Design review of the part shown in the three views and the two pictorial views. Dimensions are in mm from the part's minimum x, y and z. Coordinates: 2 decimals unless noted, no trailing zeros. Write each loop counter-clockwise with the first axis right and the second up, starting at its lowest first coordinate (ties: lowest second). Pieces come first, ordered by that corner, then holes. Notation, with made-up numbers: M 35.5,-9.5 L 73.5,-9.5 A16 cw 73.5,18.5 Z; hole C 72.25,-6.5 d2. An arc over 180 degrees is marked long. Answer as a JSON object with one key per item and string values.
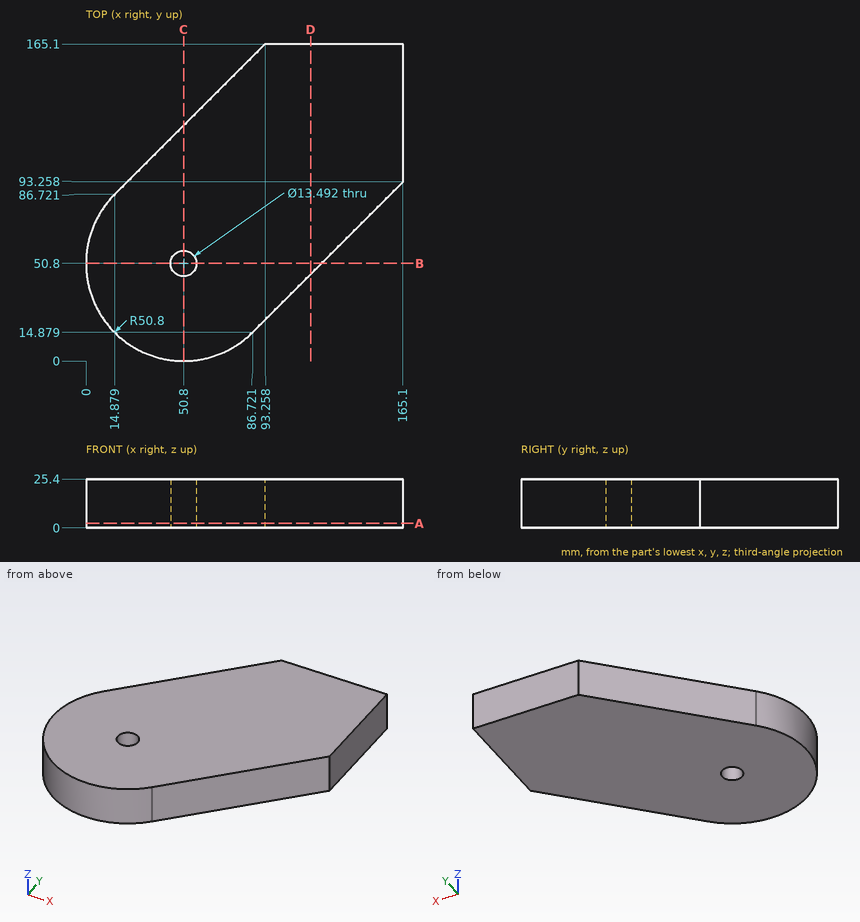
(1) For pin 1 Ø11 at (x, y) = (50.8, 50.8) entering from -Z; pin 2 Ø1 at (y, z) = (86, 8.5) entering from +X; pin 3 Ø12 at (x, z) = (62.5, 6.5) entering from +Y; pin 4 Ø10 at (x, z) = (88, 22) entering from -Y, all flat-tipped, find the tip position at first contact; note any pin that passes through.
Results list:
{"pin 1": "through", "pin 2": "x = 158.34", "pin 3": "y = 140.34", "pin 4": "y = 11.51"}
(2) Add section D-D on x = 117. Give the boundary of the cut face in (y, z).
Results list:
{"outline": "M 45.16,0 L 165.1,0 L 165.1,25.4 L 45.16,25.4 Z"}
(3) Add section A-A on z = 2.25. Give the boundary of the cut face in (x, y).
Results list:
{"outline": "M 14.88,86.72 A50.8 ccw 86.72,14.88 L 165.1,93.26 L 165.1,165.1 L 93.26,165.1 Z; hole C 50.8,50.8 d13.49"}
(4) Add section B-B on y = 50.8. Give the boundary of the cut face in (x, z).
Results list:
{"outline": "M 0,0 L 44.05,0 L 44.05,25.4 L 0,25.4 Z; M 57.55,0 L 122.64,0 L 122.64,25.4 L 57.55,25.4 Z"}
(5) Wall thickness on line 1 along Y through (x, z) = (50.8, 18) (1 decimal); line 2 along X through (y, z) = (55.5, 20.5) (1 decimal); line 3 along X through (y, z) = (75, 4.5) (1 decimal): over which ranges is each line inside the solid? List them lowest first. Write a range as from..to.
Results list:
{"line 1": "0..44.1, 57.5..122.6", "line 2": "0.2..46, 55.6..127.3", "line 3": "6.1..146.8"}
